Here's how the part is built. I have some questions about the finished solid (model axes, mm). Give positions to 0.01 mm unless a question says otherwise; leave off trailing zeros. Use one line per item in the form item = value.
```python
from build123d import *

# Parameters (mm, degrees)
SKETCH_1_W          = 442
SKETCH_1_H          = 52
EXTRUDE_1_DEPTH     = 5
SKETCH_2_R          = 2.5
CUT_EXTRUDE_1_DEPTH = 446.076397936


with BuildPart() as part:
    # 草图1 → 凸台-拉伸1 (new body)
    with BuildSketch(Plane(origin=(0, 0, 0), x_dir=(1, 0, 0), z_dir=(0, 1, 0))):
        with Locations((221, 26)):
            Rectangle(SKETCH_1_W, SKETCH_1_H)
    extrude(amount=EXTRUDE_1_DEPTH)

    # 草图2 → 切除-拉伸1 (cut, through all)
    with BuildSketch(Plane(origin=(0, 5, 0), x_dir=(1, 0, 0), z_dir=(0, 1, 0))):
        with Locations(Location((205, 8, 0), (0, 0, 270))):
            Circle(SKETCH_2_R)
        with Locations(Location((237, 8, 0), (0, 0, 90))):
            Circle(SKETCH_2_R)
        with Locations(Location((205, 44, 0), (0, 0, 90))):
            Circle(SKETCH_2_R)
        with Locations(Location((237, 44, 0), (0, 0, 270))):
            Circle(SKETCH_2_R)
        with Locations(Location((435, 44, 0), (0, 0, 270))):
            Circle(SKETCH_2_R)
        with Locations(Location((403, 44, 0), (0, 0, 90))):
            Circle(SKETCH_2_R)
        with Locations(Location((403, 8, 0), (0, 0, 270))):
            Circle(SKETCH_2_R)
        with Locations(Location((435, 8, 0), (0, 0, 90))):
            Circle(SKETCH_2_R)
        with Locations(Location((7, 44, 0), (0, 0, 90))):
            Circle(SKETCH_2_R)
        with Locations(Location((39, 44, 0), (0, 0, 270))):
            Circle(SKETCH_2_R)
        with Locations(Location((39, 8, 0), (0, 0, 90))):
            Circle(SKETCH_2_R)
        with Locations(Location((7, 8, 0), (0, 0, 270))):
            Circle(SKETCH_2_R)
    extrude(amount=-CUT_EXTRUDE_1_DEPTH, mode=Mode.SUBTRACT)


solid = part.part
```
Q1. If we mould it in two halves opening along Y, with no side actions, what happens to faces 1 (the face through (218, 5, -26)), 2 (the face through (218, 0, -26))? For each: +Y half, -Y half, draft (parallel to the pull), parting line (faces both ways), or undercut.
Result set:
face_1 = +Y half
face_2 = -Y half
Q2. Will this pin go through, and if not, where does the flat tip stop? pin 1 Ø8 at (x, z) = (403, -8) entering from -Y.
Result set:
pin_1 = 0
Q3. If I drill on line 1 along Z through (x, y) = (403, 1.5); line 2 along Z through (x, y) = (236.5, 0.65), over which ranges is the centre line in solid material (lowest first)? Write a range as from..to.
Result set:
line_1 = -52..-46.5, -41.5..-10.5, -5.5..0
line_2 = -52..-46.45, -41.55..-10.45, -5.55..0
